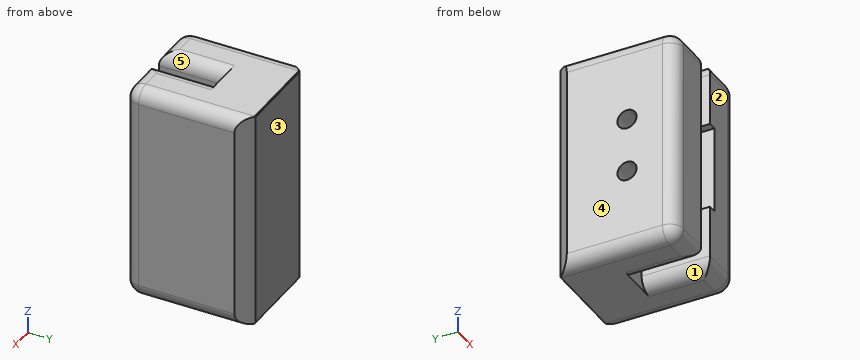
Autodesk Inventor part; units mm, degrees
ref_plane "Work Plane1" through (11.5, -22.5, 35) normal (-1, 0, 0) x (0, 0, 1)
ref_plane "YZ Plane" through (0, 0, 0) normal (1, 0, 0) x (0, 1, 0)
ref_plane "XZ Plane" through (0, 0, 0) normal (0, 1, 0) x (-1, 0, 0)
sketch "Sketch1" plane through (0, 0, 0) normal (0, 1, 0) x (-1, 0, 0)
  line L0 (-20, 40) -> (20, 40)
  line L1 (20, 40) -> (20, -40)
  line L2 (20, -40) -> (-20, -40)
  line L3 (-20, -40) -> (-20, 40)
  line L4 (-20, 40) -> (20, -40) construction
  line L5 (20, 40) -> (-20, -40) construction
  point P0 (0, 0)
  dimension "d0" = 40
  dimension "d1" = 80
extrude "Extrusion1" add sketch "Sketch1" along normal mid plane 45
sketch "Sketch2" plane through (0, -22.5, 0) normal (0, -1, 0) x (1, 0, 0)
  line L0 (20, -40) -> (-20, -40)
  line L1 (3, 40) -> (-3, 40)
  line L2 (-3, 40) -> (-3, -40)
  line L3 (-3, -40) -> (3, -40)
  line L4 (3, -40) -> (3, 40)
  line L5 (3, 40) -> (-3, -40) construction
  line L6 (-3, 40) -> (3, -40) construction
  point P0 (0, 0)
  dimension "d4" = 6
extrude "Extrusion2" cut sketch "Sketch2" against normal blind 25
chamfer "Chamfer1" distance 5 angle 45 2 edges at (20, 22.5, 0) (-20, 22.5, 0)
chamfer "Chamfer2" distance 0.3 angle 45 2 edges at (0, 22.5, 40) (0, 22.5, -40)
fillet "Fillet1" radius 5 14 edges at (20, -2.5, 40) (-20, -2.5, 40) (20, -2.5, -40) (-20, -2.5, -40) (3, -10, -40) (-3, -10, -40) (-3, -10, 40) (3, -10, 40) (-20, -22.5, 0) (-11.5, -22.5, 40) (-11.5, -22.5, -40) (11.5, -22.5, -40) (20, -22.5, 0) (11.5, -22.5, 40)
sketch "Sketch5" plane through (3, -22.5, -35) normal (-1, 0, 0) x (0, 0, 1)
  line L0 (70, 0) -> (0, 0)
  line L1 (35, 0) -> (19, 0)
  line L2 (70, 25) -> (0, 25)
  line L3 (19, 0) -> (19, 25)
  line L4 (19, 25) -> (51, 25)
  line L5 (51, 25) -> (51, 0)
  line L6 (51, 0) -> (19, 0)
  point P0 (51, 0)
  dimension "d31" = 16
  dimension "d32" = 32
extrude "Extrusion4" cut sketch "Sketch5" against normal blind 3
sketch "Sketch6" plane through (6, -22.5, -35) normal (-1, 0, 0) x (0, 0, 1)
  line L0 (19, 25) -> (51, 25)
  line L1 (19, 0) -> (19, 25)
  line L2 (51, 0) -> (19, 0)
  line L3 (51, 25) -> (51, 0)
  line L4 (19, 25) -> (51, 25)
  line L5 (35, 25) -> (35, 18)
  line L6 (35, 18) -> (25, 18)
  point P0 (35, 22.5)
  point P1 (45, 18)
  dimension "d35" = 7
  dimension "d36" = 10
hole "Hole2" at (6, -4.5, -10) at (6, -4.5, 10) direction (1, 0, 0) diameter 3.6 depth 8
ref_plane "Work Plane1" through (11.5, -22.5, 35) normal (-1, 0, 0) x (0, 0, 1)
sketch "Sketch7" plane through (11.5, -22.5, 35) normal (-1, 0, 0) x (0, 0, 1)
  line L0 (-25, 14.4204) -> (-28.1, 16.2102)
  line L1 (-28.1, 16.2102) -> (-28.1, 19.7898)
  line L2 (-28.1, 19.7898) -> (-25, 21.5796)
  line L3 (-25, 21.5796) -> (-21.9, 19.7898)
  line L4 (-21.9, 19.7898) -> (-21.9, 16.2102)
  line L5 (-21.9, 16.2102) -> (-25, 14.4204)
  line L6 (-45, 14.4204) -> (-48.1, 16.2102)
  line L7 (-48.1, 16.2102) -> (-48.1, 19.7898)
  line L8 (-48.1, 19.7898) -> (-45, 21.5796)
  line L9 (-45, 21.5796) -> (-41.9, 19.7898)
  line L10 (-41.9, 19.7898) -> (-41.9, 16.2102)
  line L11 (-41.9, 16.2102) -> (-45, 14.4204)
  line L12 (-21.9, 16.2102) -> (-21.9, 14.4204)
  line L13 (-21.9, 14.4204) -> (-28.1, 14.4204)
  line L14 (-28.1, 14.4204) -> (-28.1, 16.2102)
  line L15 (-41.9, 16.2102) -> (-41.9, 14.4204)
  line L16 (-41.9, 14.4204) -> (-48.1, 14.4204)
  line L17 (-48.1, 14.4204) -> (-48.1, 16.2102)
  point P0 (-35, 22.5)
  point P1 (-25, 18)
  point P2 (-45, 18)
  point P3 (-25, 18)
  point P4 (-45, 18)
  dimension "d52" = 6.2
  dimension "d53" = 6.2
extrude "Extrusion5" cut sketch "Sketch7" along normal blind 3.6
sketch "Sketch8" plane through (-20, -17.5, -35) normal (-1, 0, 0) x (0, 0, 1)
  circle A0 centre (25, 13) radius 1.8
  circle A1 centre (45, 13) radius 1.8
  line L0 (19, 20) -> (51, 20)
  line L1 (19, -5) -> (19, 20)
  line L2 (51, -5) -> (19, -5)
  line L3 (51, 20) -> (51, -5)
  circle A2 centre (25, 13) radius 3.5
  circle A3 centre (45, 13) radius 3.5
  point P0 (35, 17.5)
  dimension "d48" = 7
  dimension "d49" = 7
extrude "Extrusion6" cut sketch "Sketch8" against normal up to surface (23 mm away) contours A0 | A1 | A2 | A3
properties part number "SP45V1 Plastico Roldana" material "ABS Plastic"
The model under review builds one solid part; all positions refer to its coordinate system, in mm. Face numbers are marked on the shaded views. A direction names the side the tool comes from. Round coordinates to 2 decimals unless told otherwise and drop trailing zeros. Order: outer loops, then holes, each group sorted by start corner. A loop starts at its lowest first (then second) coordinate and runs counter-clockwise, first axis right, second up.
Item 1: Machinability: for the marked faces 1 and 2, which of the approach directions +Z, -Z, +X, -X, +Y, -Y give a long, thin tool a straight path to every point of the face, cutting with its end or side? Answer none if there is none.
Working result:
face 1: -Z, -Y
face 2: +Z, -Z, +X, -X, -Y
Item 2: To check wall thickness, follow probe 1 along X at (y, z) = (-7, 35); probe 2 along Z at (x, y) = (6.8, -4.5); probe 3 along Z at (x, y) = (7, -4). State the ranges of each line that lie inside material, in increasing order.
Working result:
probe 1: x = -20 to -3, 3 to 20
probe 2: z = -39.85 to -11.8, -8.2 to 8.2, 11.8 to 39.85
probe 3: z = -39.9 to -11.73, -8.27 to 8.27, 11.73 to 39.9
Item 3: Add section B-B, the plane y = -10. State the section outline as (x, z) points.
Working result:
outline: (-20, -35) arc R5 ccw to (-15, -40) - (-8, -40) arc R5 ccw to (-3, -35) - (-3, 35) arc R5 ccw to (-8, 40) - (-15, 40) arc R5 ccw to (-20, 35) - close; (3, -35) arc R5 ccw to (8, -40) - (15, -40) arc R5 ccw to (20, -35) - (20, 35) arc R5 ccw to (15, 40) - (8, 40) arc R5 ccw to (3, 35) - (3, 16) - (6, 16) - (6, -16) - (3, -16) - close
Item 4: Draft analysis for pull direction X (two halves, no side actions). For the marked faces 3, 4 and 5, state which applies: released by +X, released by -X, zero draft, split by the parting line, or undercut.
Working result:
face 3: zero draft
face 4: released by -X
face 5: undercut
Item 5: Add section A-A, the plane x = -4. State the section outline as (y, z) points.
Working result:
outline: (-22.5, -35) arc R5 ccw to (-21.5, -38) - (2.5, -38) - (2.5, -40) - (22.2, -40) - (22.5, -39.7) - (22.5, 39.7) - (22.2, 40) - (2.5, 40) - (2.5, 38) - (-21.5, 38) arc R5 ccw to (-22.5, 35) - close; hole circle Ø7 at (-4.5, -10); hole circle Ø7 at (-4.5, 10)
Item 6: For pin 1 (8 mm diameter, centred on x = -3, y = -15.5, fed in from +Z); pin 2 (5 mm diameter, centred on x = 4, y = -13.5, fed in from -Z); pin 3 (3 mm diameter, centred on y = -4.5, z = 10.5, fed in from -X), all flat-tipped, find the tip position at first contact; note any pin that passes through.
Working result:
pin 1: stops at z = 39.9
pin 2: stops at z = -39.77
pin 3: stops at x = 6
Item 7: Add section C-C, the plane z = -14.5. State the section outline as (x, y) points.
Working result:
outline: (-20, -17.5) arc R5 ccw to (-15, -22.5) - (-3, -22.5) - (-3, 2.5) - (6, 2.5) - (6, -22.5) - (15, -22.5) arc R5 ccw to (20, -17.5) - (20, 17.5) - (15, 22.5) - (-15, 22.5) - (-20, 17.5) - close
Item 8: Add section D-D, the plane y = -4.5. Count the separate pieces of the cut face and the enclosed holes in it, and give its area (3 significant figures).
Working result:
separate pieces: 4
enclosed holes: 0
area: 2,270 mm2
